from build123d import *

# Parameters (mm, degrees)
SKETCH1_W                                      = 32
SKETCH1_H                                      = 32
BOSS_EXTRUDE1_DEPTH                            = 7
CSK_FOR_M2_FLAT_HEAD_MACHINE_SCREW1_AT_2_COUNT = 2
CSK_FOR_M2_FLAT_HEAD_MACHINE_SCREW1_AT_2_PITCH = 16


with BuildPart() as part:
    # Sketch1 → Boss-Extrude1 (new body)
    with BuildSketch(Plane(origin=(0, 0, 0), x_dir=(1, 0, 0), z_dir=(0, 1, 0))):
        Rectangle(SKETCH1_W, SKETCH1_H)
    extrude(amount=BOSS_EXTRUDE1_DEPTH)

    # Sketch5 → CSK for M2 Flat Head Machine Screw1 (revolve, cut)
    with BuildSketch(Plane(origin=(-8, 7, 0), x_dir=(0, 0, 1), z_dir=(1, 0, 0))):
        Polygon((0, 0), (0, 7), (3.5, 7), (3.5, 1.732050808), (4.5, 0), align=None)
    csk_for_m2_flat_head_machine_screw1 = revolve(axis=Axis((-8, 13.35, 0), (0, -1, 0)), mode=Mode.SUBTRACT)

    # CSK for M2 Flat Head Machine Screw1 at 2: CSK for M2 Flat Head Machine Screw1 ×2
    with Locations(*[(i * CSK_FOR_M2_FLAT_HEAD_MACHINE_SCREW1_AT_2_PITCH, 0, 0) for i in range(1, CSK_FOR_M2_FLAT_HEAD_MACHINE_SCREW1_AT_2_COUNT)]):
        add(csk_for_m2_flat_head_machine_screw1, mode=Mode.SUBTRACT)


solid = part.part
Design review of the part built by this model. Coordinates are the model's own, in mm. Round coordinates to 2 decimals unless told otherwise and drop trailing zeros. Loops run counter-clockwise (first coordinate to the right, second up) from the corner with the lowest first, then second, coordinate; pieces in that order, holes last. Notation, with made-up numbers: (-10.5, 8.25) - (-3.5, 8.25) arc R14 ccw to (-3.5, 20.25) - close; hole circle Ø3 at (32, 5.25). An arc over 180 degrees is marked (long way). One line per item, written item: value. Start each with the question number.
1) Consider section B-B on x = -8. Give the boundary of the cut face in (y, z).
2) Draft analysis for pull direction Z (two halves, no side actions). For faces 1 (the flat face through (0, 3, 16)), 2 (the flat face through (16, 3, 0)), 3 (the conical face through (-4.8, 5.4, 1.6)), 4 (the flat face through (0, 3, -16)), state which applies: +Z half, -Z half, draft (parallel to the pull), parting line (faces both ways), or undercut.
3) Consider section A-A on z = 0. Give the boundary of the cut face in (x, y), then the cut area to 3 significant figures.
4) Insertion check: pin 1 Ø4 at (x, z) = (8, 0) entering from +Y; pin 2 Ø11 at (x, z) = (-8, 0) entering from +Y. Each pin has a flat end and moves straight along its axis. Give the tip position at first contact, or say it passes through.
5) Consider section C-C on y = 3. Give the boundary of the cut face in (x, z), then the cut area to 3 significant figures.
6) To check wall thickness, follow L1, parallel to X at y = 3.45, z = 0; L2, parallel to Z at x = -8, y = 3.65; L3, parallel to X at y = 0.5, z = -2. State the ranges of each line that lie inside material, in increasing order. Write a range as from..to.
7) Consider section D-D on y = 6.25. Give the boundary of the cut face in (x, z), then the cut area to 3 significant figures.
Reported:
1. outline: (0, -16) - (7, -16) - (7, -4.5) - (5.27, -3.5) - (0, -3.5) - close; (0, 3.5) - (5.27, 3.5) - (7, 4.5) - (7, 16) - (0, 16) - close
2. face 1: +Z half
2. face 2: draft
2. face 3: undercut
2. face 4: -Z half
3. outline: (-16, 0) - (-11.5, 0) - (-11.5, 5.27) - (-12.5, 7) - (-16, 7) - close; (-4.5, 0) - (4.5, 0) - (4.5, 5.27) - (3.5, 7) - (-3.5, 7) - (-4.5, 5.27) - close; (11.5, 0) - (16, 0) - (16, 7) - (12.5, 7) - (11.5, 5.27) - close
3. area: 123 mm^2
4. pin 1: passes through
4. pin 2: stops at y = 7
5. outline: (-16, -16) - (16, -16) - (16, 16) - (-16, 16) - close; hole circle Ø7 at (-8, 0); hole circle Ø7 at (8, 0)
5. area: 947 mm^2
6. L1: x = -16..-11.5, -4.5..4.5, 11.5..16
6. L2: z = -16..-3.5, 3.5..16
6. L3: x = -16..-10.87, -5.13..5.13, 10.87..16
7. outline: (-16, -16) - (16, -16) - (16, 16) - (-16, 16) - close; hole circle Ø8.13 at (-8, 0); hole circle Ø8.13 at (8, 0)
7. area: 920 mm^2
